CAD build for the part. Positions are in the model's coordinates, mm. Face numbers are marked on the shaded views. A direction names the side the tool comes from. Give positions to 0.01 mm unless a question says otherwise; leave off trailing zeros. Loops run counter-clockwise (first coordinate to the right, second up) from the corner with the lowest first, then second, coordinate; pieces in that order, holes last. Notation, with made-up numbers: (-12.5, 82.5) - (24.5, 82.5) arc R22 cw to (24.5, 109.5) - close; hole circle Ø5 at (41, -27). An arc over 180 degrees is marked (long way). Return JSON: item names as keys, results as strings.
Autodesk Inventor part; units mm, degrees
ref_plane "YZ Plane" through (0, 0, 0) normal (1, 0, 0) x (0, 1, 0)
ref_plane "XZ Plane" through (0, 0, 0) normal (0, 1, 0) x (-1, 0, 0)
ref_plane "XY Plane" through (0, 0, 0) normal (0, 0, 1) x (1, 0, 0)
sketch "Sketch1" plane through (0, 0, 0) normal (0, 1, 0) x (-1, 0, 0)
  line L0 (0, 0) -> (41.275, 0)
  line L1 (47.625, -6.35) -> (47.625, -25.4)
  arc A0 (47.625, -6.35) -> (41.275, 0) centre (41.275, -6.35) ccw
  point P0 (47.625, 0)
  dimension "d0" = 47.625
  dimension "d1" = 25.4
  dimension "d3" = 6.35
sketch "Sketch2" plane through (0, 0, 0) normal (1, 0, 0) x (0, 1, 0)
  circle A0 centre (0, 0) radius 3.175
  dimension "d2" = 6.35
sweep "Sweep1" add profiles "Sketch2" path "Sketch1"
chamfer "Chamfer1" distance 0.508 angle 45 1 edges at (0, -3.175, 0)
thread "Thread1"
chamfer "Chamfer2" distance 0.508 angle 45 1 edges at (-47.625, -3.175, -25.4)
properties part number "fc17-015_AnchorBolt" material "Steel"
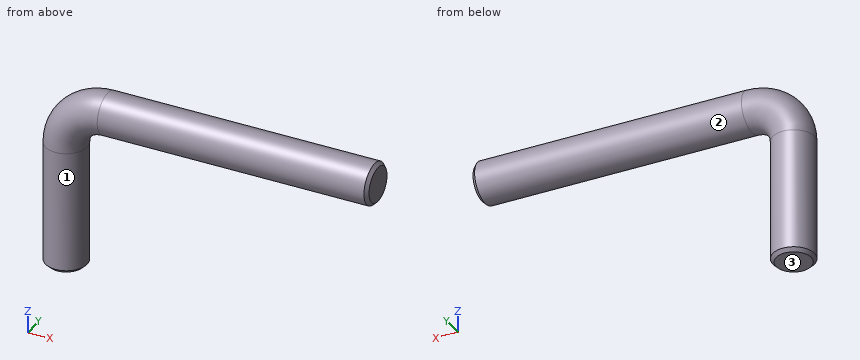
1. Drill centre lines: probe 1 along X at (y, z) = (0.25, -13.5); probe 2 along Z at (x, y) = (-24.5, 0) (3 decimals); probe 3 along Z at (x, y) = (-34, -1.5). Where is each one in solid material? Low to high.
Values follow:
{"probe 1": "x = -50.79 to -44.46", "probe 2": "z = -3.175 to 3.175", "probe 3": "z = -2.8 to 2.8"}
2. Drop flat-ended pins along their axis: P1, Ø1, axis at x = -30.5, y = 2.5, coming from the +Z side; P2, Ø2, axis at y = 2, z = -15.5, coming from the +X side. Give the stop position or say it passes through.
Values follow:
{"P1": "stops at z = 2.47", "P2": "stops at x = -44.61"}
3. Cut at C-C, the plane z = -14. Write the cut outline in (x, y) (3 decimals), plus the area to 3 significant figures.
Values follow:
{"outline": "circle Ø6.35 at (-47.625, 0)", "area": "31.7 mm²"}
4. Cut at A-A, the plane y = 0. Write the cut outline in (x, z) (3 decimals).
Values follow:
{"outline": "(-50.8, -24.892) - (-50.292, -25.4) - (-44.958, -25.4) - (-44.45, -24.892) - (-44.45, -6.35) arc R3.175 cw to (-41.275, -3.175) - (-0.508, -3.175) - (0, -2.667) - (0, 2.667) - (-0.508, 3.175) - (-41.275, 3.175) arc R9.525 ccw to (-50.8, -6.35) - close"}
5. Which spindle directions (+Z, -Z, +X, -X, +Y, -Y) get a long thin tool onto all of the face, cutting with end or side? Do the marked faces 1, 2 and 3. Say none if no direction does.
Values follow:
{"face 1": "-Z", "face 2": "+X", "face 3": "-Z, +X, -X, +Y, -Y"}
6. Cut at B-B, the plane x = -13.5. Write the cut outline in (y, z) (3 decimals), plus the area to 3 significant figures.
Values follow:
{"outline": "circle Ø6.35 at (0, 0)", "area": "31.7 mm²"}
